```python
from build123d import *

# Parameters (mm, degrees)
SKETCH1_W      = 100
SKETCH1_H      = 90
EXTRUDE1_DEPTH = 10
EXTRUDE2_DEPTH = 89.118
EXTRUDE3_DEPTH = 64.559


with BuildPart() as part:
    # Sketch1 → Extrude1 (new body)
    with BuildSketch(Plane(origin=(0, 0, 0), x_dir=(1, 0, 0), z_dir=(0, 1, 0))):
        with Locations((-40, 20)):
            Rectangle(SKETCH1_W, SKETCH1_H)
    extrude(amount=EXTRUDE1_DEPTH)

    # Sketch2 → Extrude2 (add)
    with BuildSketch(Plane(origin=(0, 10, 0), x_dir=(1, 0, 0), z_dir=(0, 1, 0))):
        Polygon((0, 0), (0, 40), (-80, 55), (-80, -15), align=None)
    extrude(amount=EXTRUDE2_DEPTH)

    # Sketch3 → Extrude3 (cut, symmetric)
    with BuildSketch(Plane.XY):
        Polygon((0, 99.118), (-80, 99.118), (-60, 91.838595315), (-60, 81.838595315), (-40, 74.559190629), (-40, 64.559190629), (-60, 71.838595315), (-60, 61.838595315), (-20, 47.279785944), (-20, 37.279785944), (-60, 51.838595315), (-60, 41.838595315), (0, 20.000381259), (0, 30.000381259), align=None)
    extrude(amount=EXTRUDE3_DEPTH, both=True, mode=Mode.SUBTRACT)


solid = part.part
```
Input: part model. Units: mm. Frame: model coordinates. A direction names the side the tool comes from. Round coordinates to 2 decimals unless told otherwise and drop trailing zeros. Loops run counter-clockwise (first coordinate to the right, second up) from the corner with the lowest first, then second, coordinate; pieces in that order, holes last. Notation, with made-up numbers: (-24.75, -31) - (21.25, -31) arc R27 cw to (21.25, -1) - close; hole circle Ø10 at (49.5, 85). An arc over 180 degrees is marked (long way). One line per item, written item: value. Start each with the question number.
(1) Section C-C, the plane z = -2. Return loops of the section in (x, y), plus the area to 3 significant figures.
(2) Section D-D, the plane y = 44. Return loops of the section in (x, z).
(3) Draft query along X for faces 1 (the flat face through (-50.14, 78.25, -19.56)), 2 (the flat face through (-80, 54, -20)), 3 (the flat face through (-60, 67, -20)). Return one class per face: +X half, -X half, draft (parallel to the pull), parting line (faces both ways), or undercut.
(4) Section A-A, the plane x = -35.5. Return loops of the section in (y, z), plus the area to 3 significant figures.
(5) Section B-B, the plane x = -49. Return loops of the section in (y, z).
(6) Contact query for flat-ended pins moving along their axis: P1, Ø5, axis at y = 14, z = -21.5, coming from the +X side; P2, Ø8, axis at y = 65.5, z = -26, coming from the +X side; P3, Ø5, axis at x = -64.5, y = 77.5, coming from the -Z side. Output: stop coordinate, or through.
(7) Ray query, line 1 (Y direction, x = -46.5, z = -43.5) (3 decimals); line 2 (Y direction, x = -43, z = -33.5); line 3 (Y direction, x = -30.5, z = -48.5). Return the intervals inside material, ascending. Write a range as [from, to].
(8) Access query for faces 4 (the flat face through (10, 5, -19)), 5 (the flat face through (-49.45, 34.13, 9.27)), 6 (the flat face through (-40.28, 54.66, -19.56)), 7 (the flat face through (-39.72, 44.457, -19.562)), 8 (the flat face through (-20, 42, -20)). Directions: +Z, -Z, +X, -X, +Y, -Y. A direction counts if a zero-diameter tool reaches every point of the face in a straight line with its end or side. Return the directions, or none.
Results below:
1. outline: (-90, 0) - (10, 0) - (10, 10) - (0, 10) - (0, 20) - (-60, 41.84) - (-60, 51.84) - (-20, 37.28) - (-20, 47.28) - (-60, 61.84) - (-60, 71.84) - (-40, 64.56) - (-40, 74.56) - (-60, 81.84) - (-60, 91.84) - (-80, 99.12) - (-80, 10) - (-90, 10) - close
1. area: 4,560 mm^2
2. outline: (-80, -55) - (-60, -51.25) - (-60, 11.25) - (-80, 15) - close; (-38.46, -47.21) - (-20, -43.75) - (-20, 3.75) - (-38.46, 7.21) - close
3. face 1: +X half
3. face 2: -X half
3. face 3: undercut
4. outline: (0, -65) - (10, -65) - (10, -46.66) - (32.92, -46.66) - (32.92, 6.66) - (10, 6.66) - (10, 25) - (0, 25) - close; (42.92, -46.66) - (52.92, -46.66) - (52.92, 6.66) - (42.92, 6.66) - close
4. area: 2,660 mm^2
5. outline: (0, -65) - (10, -65) - (10, -49.19) - (37.83, -49.19) - (37.83, 9.19) - (10, 9.19) - (10, 25) - (0, 25) - close; (47.83, -49.19) - (57.83, -49.19) - (57.83, 9.19) - (47.83, 9.19) - close; (67.83, -49.19) - (77.83, -49.19) - (77.83, 9.19) - (67.83, 9.19) - close
6. P1: x = 0
6. P2: x = -40
6. P3: z = -52.56
7. line 1: [0, 36.925], [46.925, 56.925], [66.925, 76.925]
7. line 2: [0, 35.65], [45.65, 55.65], [65.65, 75.65]
7. line 3: [0, 10]
8. face 4: +Z, -Z, +X, +Y, -Y
8. face 5: +Z, +X, +Y
8. face 6: +Z, -Z, +X
8. face 7: +Z, -Z
8. face 8: +Z, -Z, +X, +Y
